```python
from build123d import *

# Parameters (mm, degrees)
F0_R     = 1.1
F1_DEPTH = 10
F2_R     = 1.1
F3_DEPTH = 6
F4_R     = 1.1
F5_DEPTH = 2
F6_R     = 15
F6_R_2   = 10
F7_DEPTH = 9
F8_W     = 28
F8_H     = 8
F9_DEPTH = 9.8


with BuildPart() as f1:
    # F0 (on Front) → F1 (new body)
    with BuildSketch(Plane.XZ):
        with BuildLine():
            Line((-18, -20), (18, -20))
            ThreePointArc((18, -20), (19.414214, -19.414214), (20, -18))
            Line((20, -18), (20, 18))
            ThreePointArc((20, 18), (19.414214, 19.414214), (18, 20))
            Line((18, 20), (-18, 20))
            ThreePointArc((-18, 20), (-19.414214, 19.414214), (-20, 18))
            Line((-20, 18), (-20, -18))
            ThreePointArc((-20, -18), (-19.414214, -19.414214), (-18, -20))
        make_face()
        with Locations((-17.25, -17.25)):
            Circle(F0_R, mode=Mode.SUBTRACT)
        with Locations((17.25, -17.25)):
            Circle(F0_R, mode=Mode.SUBTRACT)
        with Locations((-17.25, 17.25)):
            Circle(F0_R, mode=Mode.SUBTRACT)
        with Locations((17.25, 17.25)):
            Circle(F0_R, mode=Mode.SUBTRACT)
    extrude(amount=F1_DEPTH)

    # F2 (on face) → F3 (cut)
    with BuildSketch(Plane.XZ.offset(10)):
        with BuildLine():
            Line((-18, -20), (-15, -20))
            Line((-15, -20), (-15, -17))
            ThreePointArc((-15, -17), (-15.585786, -15.585786), (-17, -15))
            Line((-17, -15), (-20, -15))
            Line((-20, -15), (-20, -18))
            ThreePointArc((-20, -18), (-19.414214, -19.414214), (-18, -20))
        make_face()
        with Locations((-17.25, -17.25)):
            Circle(F2_R, mode=Mode.SUBTRACT)
        with BuildLine():
            Line((-20, 18), (-20, 15))
            Line((-20, 15), (-17, 15))
            ThreePointArc((-17, 15), (-15.585786, 15.585786), (-15, 17))
            Line((-15, 17), (-15, 20))
            Line((-15, 20), (-18, 20))
            ThreePointArc((-18, 20), (-19.414214, 19.414214), (-20, 18))
        make_face()
        with Locations((-17.25, 17.25)):
            Circle(F2_R, mode=Mode.SUBTRACT)
        with BuildLine():
            Line((17, 15), (20, 15))
            Line((20, 15), (20, 18))
            ThreePointArc((20, 18), (19.414214, 19.414214), (18, 20))
            Line((18, 20), (15, 20))
            Line((15, 20), (15, 17))
            ThreePointArc((15, 17), (15.585786, 15.585786), (17, 15))
        make_face()
        with Locations((17.25, 17.25)):
            Circle(F2_R, mode=Mode.SUBTRACT)
        with BuildLine():
            Line((15, -17), (15, -20))
            Line((15, -20), (18, -20))
            ThreePointArc((18, -20), (19.414214, -19.414214), (20, -18))
            Line((20, -18), (20, -15))
            Line((20, -15), (17, -15))
            ThreePointArc((17, -15), (15.585786, -15.585786), (15, -17))
        make_face()
        with Locations((17.25, -17.25)):
            Circle(F2_R, mode=Mode.SUBTRACT)
    extrude(amount=-F3_DEPTH, mode=Mode.SUBTRACT)

    # F4 (on face) → F5 (cut)
    with BuildSketch(Plane(origin=(0, 0, 0), x_dir=(-1, 0, 0), z_dir=(0, 1, 0))):
        with BuildLine():
            Line((-18, -20), (-15, -20))
            Line((-15, -20), (-15, -17))
            ThreePointArc((-15, -17), (-15.585786, -15.585786), (-17, -15))
            Line((-17, -15), (-20, -15))
            Line((-20, -15), (-20, -18))
            ThreePointArc((-20, -18), (-19.414214, -19.414214), (-18, -20))
        make_face()
        with Locations((-17.25, -17.25)):
            Circle(F4_R, mode=Mode.SUBTRACT)
        with BuildLine():
            Line((-15, 17), (-15, 20))
            Line((-15, 20), (-18, 20))
            ThreePointArc((-18, 20), (-19.414214, 19.414214), (-20, 18))
            Line((-20, 18), (-20, 15))
            Line((-20, 15), (-17, 15))
            ThreePointArc((-17, 15), (-15.585786, 15.585786), (-15, 17))
        make_face()
        with Locations((-17.25, 17.25)):
            Circle(F4_R, mode=Mode.SUBTRACT)
        with BuildLine():
            Line((17, 15), (20, 15))
            Line((20, 15), (20, 18))
            ThreePointArc((20, 18), (19.414214, 19.414214), (18, 20))
            Line((18, 20), (15, 20))
            Line((15, 20), (15, 17))
            ThreePointArc((15, 17), (15.585786, 15.585786), (17, 15))
        make_face()
        with Locations((17.25, 17.25)):
            Circle(F4_R, mode=Mode.SUBTRACT)
        with BuildLine():
            Line((20, -15), (17, -15))
            ThreePointArc((17, -15), (15.585786, -15.585786), (15, -17))
            Line((15, -17), (15, -20))
            Line((15, -20), (18, -20))
            ThreePointArc((18, -20), (19.414214, -19.414214), (20, -18))
            Line((20, -18), (20, -15))
        make_face()
        with Locations((17.25, -17.25)):
            Circle(F4_R, mode=Mode.SUBTRACT)
    extrude(amount=-F5_DEPTH, mode=Mode.SUBTRACT)

    # F6 (on face) → F7 (cut)
    with BuildSketch(Plane.XZ.offset(10)):
        with Locations((3, 0)):
            Circle(F6_R)
        with Locations((3, 0)):
            Circle(F6_R_2, mode=Mode.SUBTRACT)
    extrude(amount=-F7_DEPTH, mode=Mode.SUBTRACT)

    # F8 (on face) → F9 (cut)
    with BuildSketch(Plane(origin=(0, 0, -20), x_dir=(1, 0, 0), z_dir=(0, 0, -1))):
        with Locations((0, 5)):
            Rectangle(F8_W, F8_H)
    extrude(amount=-F9_DEPTH, mode=Mode.SUBTRACT)


solid = f1.part
```
Can you work these out from the model? Positions are in its coordinate system, mm. A direction names the side the tool comes from. Give positions to 0.01 mm unless a question says otherwise; leave off trailing zeros. Loops run counter-clockwise (first coordinate to the right, second up) from the corner with the lowest first, then second, coordinate; pieces in that order, holes last. Notation, with made-up numbers: M 4,29.5 L 47,29.5 A20 cw 47,52.5 Z; hole C -36,37 d5. An arc over 180 degrees is marked long. Use one line per item in the form item = value. Start each with the question number.
(1) Please list where these lines run through material, in increasing order: line 1 (X direction, y = -5.5, z = -14); line 2 (Z direction, x = -16.5, y = -2.75); line 3 (Z direction, x = 3, y = -4.25).
(2) I'm going to push flat-ended pins straight in: P1, Ø1.3, axis at x = 17.25, z = -17.25, coming from the +Y side; P2, Ø3.5, axis at x = 17.25, z = 17.25, coming from the +Y side; P3, Ø0.6, axis at y = -1, z = 18.5, coming from the +X side; P4, Ø0.9, axis at x = -18.5, y = -6.5, coming from the -Z side. Where does each tip first touch, or does it pass through?
(3) On a 3-axis mill with a long thin cutter (end or side, diameter ignored), from which of +Z, -Z, +X, -X, +Y, -Y can I reach the whole of each face in a straight line? I mean faces 1 (the flat face through (15, -7, 19)), 2 (the flat face through (19, -1, 15)), 3 (the flat face through (15, -1, -19)), 4 (the cylindrical face through (-15.6, -0.99, -15.57)). Say none if no direction works.
(4) I want a section at C-C, the plane z = 0. Write out the boundary of the cut face in (x, y).
(5) Thinking about a two-plate mould opening in Z: for faces 5 (the cylindrical face through (1.047, -5.563, 14.872)), 6 (the flat face through (-19, -7, 15)), 7 (the cylindrical face through (19.4, -2.99, -19.43)), 8 (the flat face through (17, -4, -19)), which applies, released by +Z, released by -Z, zero draft, split by the parting line, or undercut?
(6) I want a section at A-A, the plane x = 3. Write out the boundary of the cut face in (y, z).
(7) I want a section at D-D, the plane x = -11.5. Write out the boundary of the cut face in (y, z), and give its area (3 significant figures).
Worked out:
q1.line_1 = -20 to -14, 14 to 20
q1.line_2 = -20 to -18.05, -16.45 to 16.45, 18.05 to 20
q1.line_3 = -10 to 10, 15 to 20
q2.P1 = through
q2.P2 = -2
q2.P3 = 15
q2.P4 = -15
q3.face_1 = +Z, +X, -Y
q3.face_2 = +Z, +X, +Y
q3.face_3 = -Z, +X, +Y
q3.face_4 = -Z, -X, +Y
q4.outline = M -20,-10 L -12,-10 L -12,-1 L -7,-1 L -7,-10 L 13,-10 L 13,-1 L 18,-1 L 18,-10 L 20,-10 L 20,0 L -20,0 Z
q5.face_5 = undercut
q5.face_6 = released by +Z
q5.face_7 = released by -Z
q5.face_8 = zero draft
q6.outline = M -10,-20 L -9,-20 L -9,-15 L -10,-15 Z; M -10,-10 L -1,-10 L -1,-20 L 0,-20 L 0,20 L -10,20 L -10,15 L -1,15 L -1,10 L -10,10 Z
q7.outline = M -10,-20 L -9,-20 L -9,-10.2 L -1,-10.2 L -1,-20 L 0,-20 L 0,20 L -10,20 L -10,3.84 L -1,3.84 L -1,-3.84 L -10,-3.84 Z
q7.area = 252 mm²
